Read the model definition and answer for the solid it produces. Units are mm, in the model's axes. A direction names the side the tool comes from. Round coordinates to 2 decimals unless told otherwise and drop trailing zeros. Loops run counter-clockwise (first coordinate to the right, second up) from the corner with the lowest first, then second, coordinate; pieces in that order, holes last. Notation, with made-up numbers: (53.25, 85.5) -> (110.25, 85.5) arc R23 ccw to (110.25, 111.5) -> close; hole circle Ø7 at (59.5, 54.25). An arc over 180 degrees is marked (long way). Put each result on its own line as item: value.
from build123d import *


with BuildPart() as part:
    # Sketch1 → Revolve-Thin1 (revolve)
    with BuildSketch(Plane.XY, mode=Mode.PRIVATE) as revolve_thin1_sk:
        with BuildLine():
            Line((12.954, -1.905), (12.954, -10.541))
            Line((12.954, -10.541), (7.196666667, 0.254))
            Line((7.196666667, 0.254), (10.795, 0.254))
            ThreePointArc((10.795, 0.254), (12.321643541, -0.378356459), (12.954, -1.905))
        make_face()
        with BuildLine():
            Line((12.446, -1.905), (12.446, -8.509))
            Line((12.446, -8.509), (8.043333333, -0.254))
            Line((8.043333333, -0.254), (10.795, -0.254))
            ThreePointArc((10.795, -0.254), (11.962433296, -0.737566704), (12.446, -1.905))
        make_face(mode=Mode.SUBTRACT)
    revolve(revolve_thin1_sk.sketch.rotate(Axis((0, 31.836101695, 0), (0, -1, 0)), 90), axis=Axis((0, 31.836101695, 0), (0, -1, 0)))


solid = part.part
Item 1: The part is cut by section D-D (y = -9). Determine the outline of the cut face in (x, z).
Derived:
outline: circle Ø25.91 at (0, 0); hole circle Ø24.26 at (0, 0)
Item 2: Which of the six approach directions +Z, -Z, +X, -X, +Y, -Y give full straight-line access (tool end or side, diameter ignored) to faces 4 (the flat face through (-8, -0.254, 2)), 5 (the conical face through (-2.44, -1.47, 7.74))?
Derived:
face 4: none
face 5: -Y
Item 3: The part is cut by section B-B (x = 0). Determine the outline of the cut face in (y, z) (3 decimals), then the cut area to 3 significant figures.
Derived:
outline: (-10.541, -12.954) -> (-1.905, -12.954) arc R2.159 ccw to (0.254, -10.795) -> (0.254, -7.197) -> close; (-10.541, 12.954) -> (0.254, 7.197) -> (0.254, 10.795) arc R2.159 ccw to (-1.905, 12.954) -> close; hole (-8.509, -12.446) -> (-1.905, -12.446) arc R1.651 ccw to (-0.254, -10.795) -> (-0.254, -8.043) -> close; hole (-8.509, 12.446) -> (-0.254, 8.043) -> (-0.254, 10.795) arc R1.651 ccw to (-1.905, 12.446) -> close
area: 25.0 mm^2
Item 4: The part is cut by section C-C (y = -6). Determine the outline of the cut face in (x, z), then the cut area to 3 significant figures.
Derived:
outline: circle Ø25.91 at (0, 0); circle Ø22.22 at (0, 0); hole circle Ø24.89 at (0, 0); hole circle Ø21.06 at (0, 0)
area: 79.7 mm^2
Item 5: For a pull along Z with two mould halves and no side action, classify faces 1 (the cylindrical face through (11.042, -5.253, 5.743)), 2 (the flat face through (7.05, 0.254, -2.25)), 3 (the cylindrical face through (12.646, -6.283, -2.808)) as pulls with the +Z half, pulls with the -Z half, needs draft (parallel to the pull), parting line crosses it, or undercut.
Derived:
face 1: undercut
face 2: needs draft
face 3: parting line crosses it
Item 6: The part is cut by section A-A (z = 0). Determine the outline of the cut face in (x, y) (3 decimals).
Derived:
outline: (-12.954, -10.541) -> (-7.197, 0.254) -> (-10.795, 0.254) arc R2.159 ccw to (-12.954, -1.905) -> close; (7.197, 0.254) -> (12.954, -10.541) -> (12.954, -1.905) arc R2.159 ccw to (10.795, 0.254) -> close; hole (-12.446, -8.509) -> (-8.043, -0.254) -> (-10.795, -0.254) arc R1.651 ccw to (-12.446, -1.905) -> close; hole (8.043, -0.254) -> (12.446, -8.509) -> (12.446, -1.905) arc R1.651 ccw to (10.795, -0.254) -> close
Item 7: Flat-ended cylindrical pins translate along their axes: pin 1 Ø3 at (x, y) = (9.5, -5) entering from +Z; pin 2 Ø1.5 at (x, y) = (2.5, -4) entering from -Z; pin 3 Ø4 at (x, z) = (-5.5, 5) entering from -Y. Find the tip coordinate at first contact, or state that the pin passes through.
Derived:
pin 1: stops at z = 10.19
pin 2: stops at z = -12.84
pin 3: stops at y = -3.94
Item 8: Find the intervals of material crossed by line 1 along Z through (x, y) = (3.5, -7); line 2 along X through (y, z) = (-5, -2.25); line 3 along X through (y, z) = (-2, -1), in increasing order.
Derived:
line 1: z = -12.47 to -11.94, -11.1 to -10.5, 10.5 to 11.1, 11.94 to 12.47
line 2: x = -12.76 to -12.24, -10.33 to -9.74, 9.74 to 10.33, 12.24 to 12.76
line 3: x = -12.92 to -12.41, -8.92 to -8.34, 8.34 to 8.92, 12.41 to 12.92
